The model under review builds one solid part; all positions refer to its coordinate system, in mm. A direction names the side the tool comes from. Round coordinates to 2 decimals unless told otherwise and drop trailing zeros. Write each loop counter-clockwise with the first axis right and the second up, starting at its lowest first coordinate (ties: lowest second). Pieces come first, ordered by that corner, then holes. Notation, with made-up numbers: M 83.5,14 L 91.5,14 A11 cw 91.5,35 Z; hole C -30,35.25 d2. An arc over 180 degrees is marked long. One line per item, written item: value. Start each with the question number.
1) Take a section at A-A, the plane z = 0. Write out the cut boundary in (x, y), and give its area (3 significant figures).
2) Take a section at B-B, the plane x = 0. Write out the cut boundary in (y, z).
3) Wall thickness on probe 1 along X at (y, z) = (-80.25, 0); probe 2 along X at (y, z) = (4, 0); probe 3 along Y at (x, z) = (-11, -19): over which ranges is each line inside the solid? List them lowest first.
4) Tool access review of faces 4 (the face through (-8.054, -82.395, 1.788)), 5 (the face through (-8.48, -36.98, -20.45)), 6 (the face through (-6.876, 4.93, -8.967)): name each direction out of +Z, -Z, +X, -X, +Y, -Y from which nothing blocks a thin tool from reaching the whole face with its end or side.
5) Take a section at D-D, the plane z = -19. Write out the cut boundary in (x, y).
6) For P1, Ø2, axis at y = -69, z = -7.5, coming from the -X side; P2, Ø11.5, axis at x = -3, z = -3, coming from the +Y side; P3, Ø2, axis at y = -79, z = -8, coming from the -X side, all flat-tipped, find the tip position at first contact; note any pin that passes through.
7) Mouldability with a two-part tool opening along X and no side actions: class faces 1 (the face through (-10, 0, -10)), 2 (the face through (-7.789, 4.93, -10.158)), 3 (the face through (0, 0, 0)) as +X half, -X half, draft (parallel to the pull), parting line (faces both ways), or undercut.
8) Take a section at C-C, the plane y = -38. Write out the cut boundary in (x, z), and give its area (3 significant figures).
from build123d import *

# Parameters (mm, degrees)
SKETCH1_R           = 12.8
SKETCH1_R_2         = 11.3
BOSS_EXTRUDE1_DEPTH = 10
SKETCH2_R           = 22.139080492
BOSS_EXTRUDE2_DEPTH = 75
SKETCH3_R           = 11.25
SKETCH3_R_2         = 8.25
BOSS_EXTRUDE3_DEPTH = 15


with BuildPart() as part:
    # Sketch1 → Boss-Extrude1 (new body)
    with BuildSketch(Plane(origin=(0, 0, 0), x_dir=(1, 0, 0), z_dir=(0, 1, 0))):
        with Locations(Location((0, 0, 0), (0, 0, 270))):
            Circle(SKETCH1_R)
        with Locations(Location((0, 0, 0), (0, 0, 270))):
            Circle(SKETCH1_R_2, mode=Mode.SUBTRACT)
    extrude(amount=BOSS_EXTRUDE1_DEPTH)

    # Sketch2 → Boss-Extrude2 (add)
    with BuildSketch(Plane.XZ):
        with Locations(Location((0, 0, 0), (0, 0, 270))):
            Circle(SKETCH2_R)
    extrude(amount=BOSS_EXTRUDE2_DEPTH)

    # Sketch3 → Boss-Extrude3 (add)
    with BuildSketch(Plane.XZ.offset(75)):
        with Locations(Location((0, 0, 0), (0, 0, 270))):
            Circle(SKETCH3_R)
        with Locations(Location((0, 0, 0), (0, 0, 270))):
            Circle(SKETCH3_R_2, mode=Mode.SUBTRACT)
    extrude(amount=BOSS_EXTRUDE3_DEPTH)


solid = part.part
Checked values:
1. outline: M -22.14,-75 L -11.25,-75 L -11.25,-90 L -8.25,-90 L -8.25,-75 L 8.25,-75 L 8.25,-90 L 11.25,-90 L 11.25,-75 L 22.14,-75 L 22.14,0 L 12.8,0 L 12.8,10 L 11.3,10 L 11.3,0 L -11.3,0 L -11.3,10 L -12.8,10 L -12.8,0 L -22.14,0 Z
1. area: 3,440 mm2
2. outline: M -90,-11.25 L -75,-11.25 L -75,-22.14 L 0,-22.14 L 0,-12.8 L 10,-12.8 L 10,-11.3 L 0,-11.3 L 0,11.3 L 10,11.3 L 10,12.8 L 0,12.8 L 0,22.14 L -75,22.14 L -75,11.25 L -90,11.25 L -90,8.25 L -75,8.25 L -75,-8.25 L -90,-8.25 Z
3. probe 1: x = -11.25 to -8.25, 8.25 to 11.25
3. probe 2: x = -12.8 to -11.3, 11.3 to 12.8
3. probe 3: y = -75 to 0
4. face 4: -Y
4. face 5: +Y, -Y
4. face 6: +Y
5. outline: M -11.36,-75 L 11.36,-75 L 11.36,0 L -11.36,0 Z
6. P1: stops at x = -21.16
6. P2: stops at y = 0
6. P3: stops at x = -8.81
7. face 1: draft
7. face 2: parting line
7. face 3: undercut
8. outline: C 0,0 d44.28
8. area: 1,540 mm2
